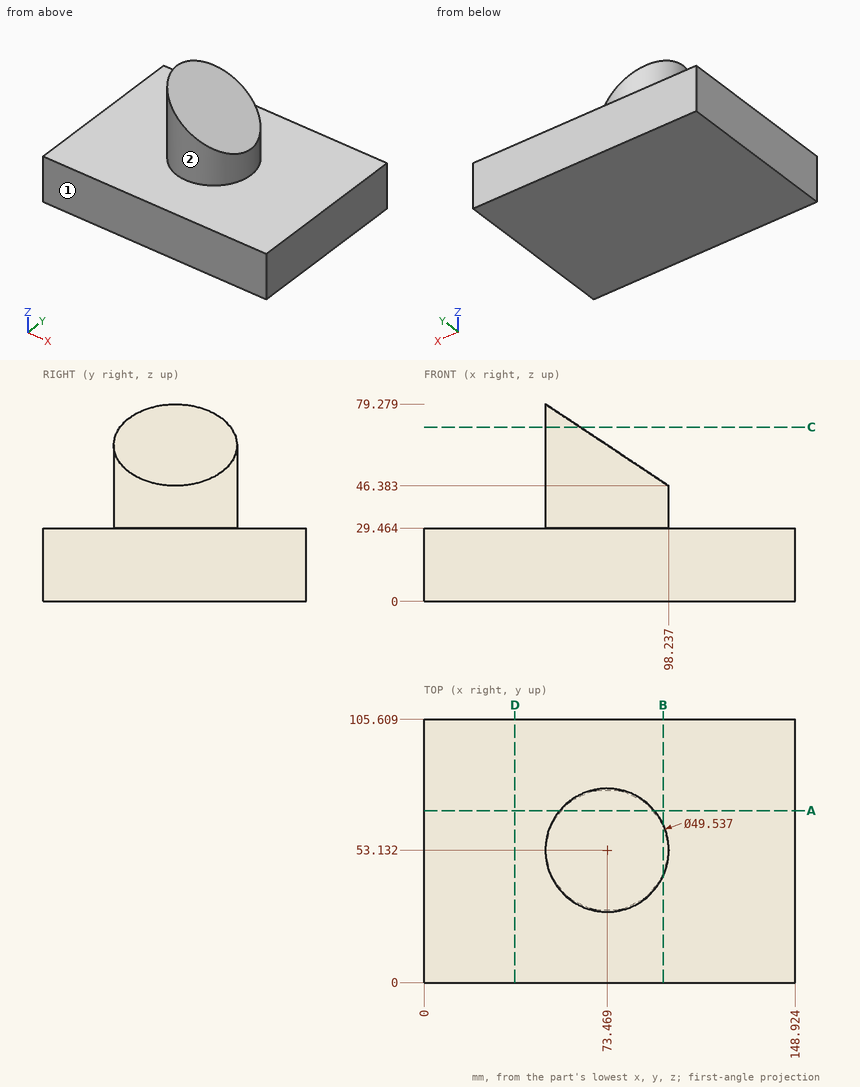
Check sheet for the drawn part. Datum: minimum x, y, z corner. Units: mm. A direction names the side the tool comes from. Round coordinates to 2 decimals unless told otherwise and drop trailing zeros. Order: outer loops, then holes, each group sorted by start corner. A loop starts at its lowest first (then second) coordinate and runs counter-clockwise, first axis right, second up. Notation, with made-up numbers: (-40, 23) -> (-25, 23) arc R24 cw to (-25, 62) -> close; hole circle Ø2 at (-18, -4.5). An arc over 180 degrees is marked (long way). Put each result on its own line as item: value.
1) Set-up check for the marked faces 1 and 2: record each of +Z, -Z, +X, -X, +Y, -Y from which the full face is reachable in a straight line by a thin tool's end or side.
Final values:
face 1: +Z, -Z, +X, -X, -Y
face 2: +Z
2) Section check C-C (z = 70). Record the cut outline in (x, y) (1 decimal).
Final values:
outline: (62.7, 30.8) -> (62.7, 75.4) arc R24.8 ccw to start
3) Depth check by flat-ended pin: pin 1 (3 mm diameter, centred on y = 70, z = 32.5, fed in from +X); pin 2 (1.5 mm diameter, centred on x = 102, y = 83.5, fed in from +Z); pin 3 (6 mm diameter, centred on y = 59.5, z = 52.5, fed in from +X) (1 decimal). Enter the tip coordinate at first touch or a pass-through.
Final values:
pin 1: stops at x = 92.89
pin 2: stops at z = 29.46
pin 3: stops at x = 93.5
4) Material ranges on line 1 (Z direction, x = 102.5, y = 15.5); line 2 (Z direction, x = 92.5, y = 44.5) (1 decimal); line 3 (X direction, y = 45, z = 63.5) (1 decimal), recorded low to high.
Final values:
line 1: z = 0 to 29.46
line 2: z = 0 to 50.2
line 3: x = 50.1 to 72.5
5) Section check B-B (x = 96). Record the cut outline in (y, z) (1 decimal).
Final values:
outline: (0, 0) -> (105.6, 0) -> (105.6, 29.5) -> (63.4, 29.5) -> (63.4, 47.9) -> (42.8, 47.9) -> (42.8, 29.5) -> (0, 29.5) -> close
6) Section check D-D (x = 36.5). Record the cut outline in (y, z), then the cut area to 3 significant figures.
Final values:
outline: (0, 0) -> (105.61, 0) -> (105.61, 29.46) -> (0, 29.46) -> close
area: 3,110 mm^2
7) Section check A-A (y = 69). Record the cut outline in (x, z), then the cut area to 3 significant figures.
Final values:
outline: (0, 0) -> (148.92, 0) -> (148.92, 29.46) -> (92.49, 29.46) -> (92.49, 50.2) -> (54.45, 75.46) -> (54.45, 29.46) -> (0, 29.46) -> close
area: 5,660 mm^2
